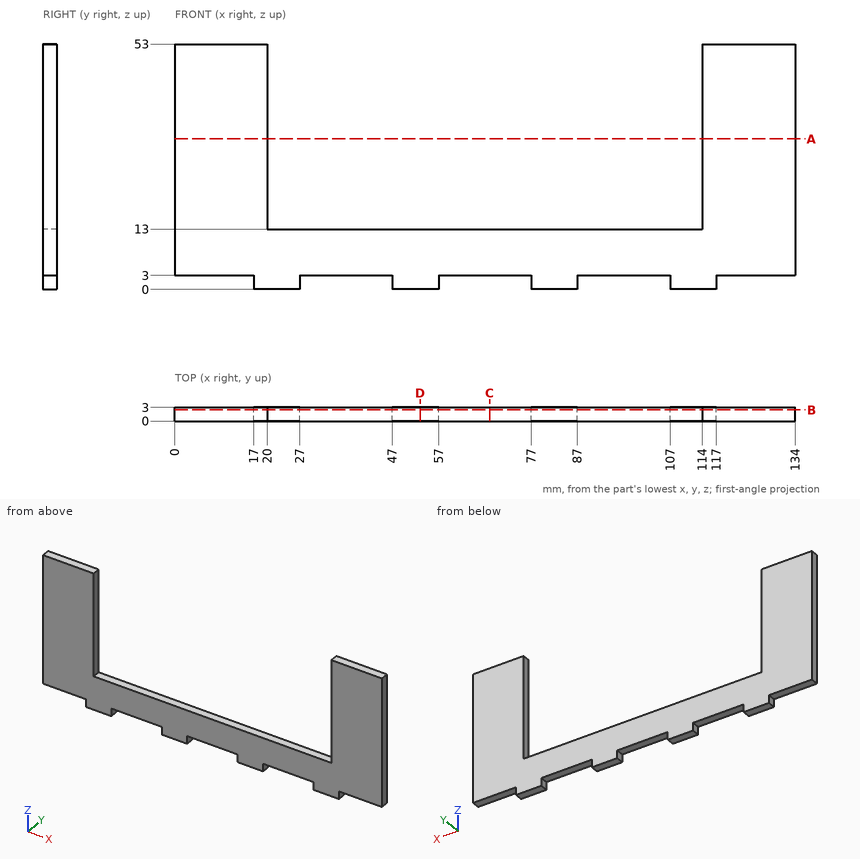
Here's the drawing with two shaded views (mm, measured from the low corner). I have some questions. Coordinates: 2 decimals unless noted, no trailing zeros. Write each loop counter-clockwise with the first axis right and the second up, starting at its lowest first coordinate (ties: lowest second). Pieces come first, ordered by that corner, then holes. Notation, with made-up numbers: M 68,31.5 L 84,31.5 A27 cw 84,50.5 Z; hole C 80.5,38.5 d6. An arc over 180 degrees is marked long. Answer as CSV lines item,"result". Start each with the question number.
1) I want a section at D-D, the plane x = 53. Please give me the cut outline in (y, z).
2) Please list where these lines run through material, in increasing order: line 1 (X direction, y = 2.55, z = 34.5); line 2 (Z direction, x = 73, y = 0.7); line 3 (Z direction, x = 56.5, y = 0.95). Write a range as from..to.
3) For P1, Ø1.5, axis at y = 1, z = 2, coming from the +X side; P2, Ø1.5, axis at x = 10.5, y = 1, coming from the -Z side; P3, Ø1, axis at x = 88, y = 2, coming from the +Z side, each with a flat end and sliding along its axis, tell me the tip position at first contact or that it passes through.
4) I want a section at A-A, the plane z = 32.5. Please give me the cut outline in (x, y), and give its area (3 significant figures).
5) I want a section at B-B, the plane y = 2.45. Please give me the cut outline in (x, z), and give its area (3 significant figures).
6) I want a section at C-C, the plane x = 68. Please give me the cut outline in (y, z), and give its area (3 significant figures).
Data:
1,outline,"M 0,0 L 3,0 L 3,13 L 0,13 Z"
2,line 1,"x = 0..20, 114..134"
2,line 2,"z = 3..13"
2,line 3,"z = 0..13"
3,P1,"stops at x = 117"
3,P2,"stops at z = 3"
3,P3,"stops at z = 13"
4,outline,"M 0,0 L 20,0 L 20,3 L 0,3 Z; M 114,0 L 134,0 L 134,3 L 114,3 Z"
4,area,"120 mm^2"
5,outline,"M 0,3 L 17,3 L 17,0 L 27,0 L 27,3 L 47,3 L 47,0 L 57,0 L 57,3 L 77,3 L 77,0 L 87,0 L 87,3 L 107,3 L 107,0 L 117,0 L 117,3 L 134,3 L 134,53 L 114,53 L 114,13 L 20,13 L 20,53 L 0,53 Z"
5,area,"3,060 mm^2"
6,outline,"M 0,3 L 3,3 L 3,13 L 0,13 Z"
6,area,"30.0 mm^2"
